The drawing under review shows one solid part. Ordinate dimensions are in mm from its lowest x, y, z. Coordinates: 2 decimals unless noted, no trailing zeros. Order: outer loops, then holes, each group sorted by start corner. A loop starts at its lowest first (then second) coordinate and runs counter-clockwise, first axis right, second up. Notation, with made-up numbers: (63.5, 12) -> (91.5, 12) arc R17 ccw to (91.5, 40) -> close; hole circle Ø1 at (45, -2.5). An arc over 180 degrees is marked (long way). Use one line per item in the form item = value.
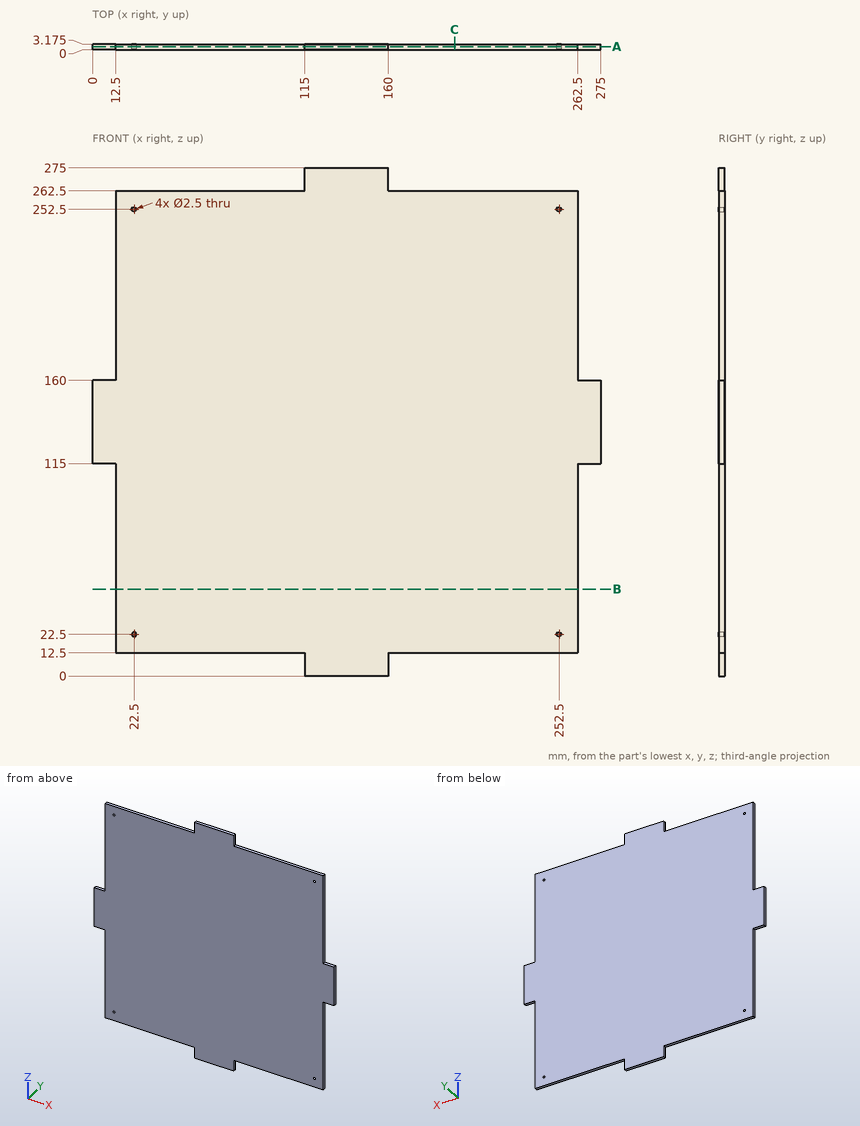
Item 1: Clearance check with flat-ended pins moving along their axes: pin 1 (2 mm diameter, centred on x = 22.5, z = 252.5, fed in from +Y); pin 2 (1 mm diameter, centred on x = 40.5, y = 2, fed in from +Z); pin 3 (1.6 mm diameter, centred on x = 5, y = 1, fed in from +Z); pin 4 (1 mm diameter, centred on y = 2.5, z = 89, fed in from -X). State where each tip first meets the part, or that it passes through.
Results found:
pin_1 = through
pin_2 = 262.5
pin_3 = 160
pin_4 = 12.5
Item 2: We need section B-B (z = 47). Write out the cut boundary in (x, y) (3 decimals).
Results found:
outline = (12.5, 0) -> (262.5, 0) -> (262.5, 3.175) -> (12.5, 3.175) -> close
Item 3: To check wall thickness, follow L1, parallel to X at y = 1.25, z = 22.5; L2, parallel to X at y = 2.1, z = 73. State the ranges of each line that lie inside material, in increasing order. Write a range as from..to.
Results found:
L1 = 12.5..21.25, 23.75..251.25, 253.75..262.5
L2 = 12.5..262.5
Item 4: We need section A-A (y = 1.75). Write out the cut boundary in (x, z).
Results found:
outline = (0, 115) -> (12.5, 115) -> (12.5, 12.5) -> (115, 12.5) -> (115, 0) -> (160, 0) -> (160, 12.5) -> (262.5, 12.5) -> (262.5, 115) -> (275, 115) -> (275, 160) -> (262.5, 160) -> (262.5, 262.5) -> (160, 262.5) -> (160, 275) -> (115, 275) -> (115, 262.5) -> (12.5, 262.5) -> (12.5, 160) -> (0, 160) -> close; hole circle Ø2.5 at (22.5, 22.5); hole circle Ø2.5 at (22.5, 252.5); hole circle Ø2.5 at (252.5, 22.5); hole circle Ø2.5 at (252.5, 252.5)
Item 5: We need section C-C (x = 196). Write out the cut boundary in (y, z) (3 decimals), plus the area to 3 significant figures.
Results found:
outline = (0, 12.5) -> (3.175, 12.5) -> (3.175, 262.5) -> (0, 262.5) -> close
area = 794 mm²
